from build123d import *

# Parameters (mm, degrees)
SKETCH_1_W          = 40.75
SKETCH_1_H          = 20.2
EXTRUDE_1_DEPTH     = 20.65
SHELL_1_T           = -1.65
SKETCH_2_W          = 40.75
SKETCH_2_H          = 20.2
EXTRUDE_2_DEPTH     = 1
EXTRUDE_3_DEPTH     = 1.23
SKETCH_4_R          = 3.95
SKETCH_4_R_2        = 0.8
EXTRUDE_4_DEPTH     = 5
EXTRUDE_5_DEPTH     = 2
SKETCH_6_R          = 2.9
SKETCH_6_R_2        = 2.4
EXTRUDE_6_DEPTH     = 4
SKETCH_7_W          = 38.95
SKETCH_7_H          = 18.4
CUT_EXTRUDE_2_DEPTH = 2.6
SKETCH_9_R          = 1.4
EXTRUDE_7_DEPTH     = 17.05
CUT_EXTRUDE_START   = -19.28
SKETCH_8_R          = 1
CUT_EXTRUDE_3_DEPTH = 19.28


with BuildPart() as part:
    # Эскиз1 → Бобышка-Вытянуть1 (new body)
    with BuildSketch(Plane(origin=(0, 0, 0), x_dir=(1, 0, 0), z_dir=(0, 1, 0))):
        Rectangle(SKETCH_1_W, SKETCH_1_H)
    extrude(amount=EXTRUDE_1_DEPTH)

    # Оболочка1
    shell_1_openings = [part.faces().sort_by_distance(p)[0] for p in [
        (0, 20.65, 0),
        (0, 0, 0),
    ]]
    offset(amount=SHELL_1_T, openings=shell_1_openings, kind=Kind.INTERSECTION)

    # Эскиз2 → Бобышка-Вытянуть2 (add)
    with BuildSketch(Plane(origin=(0, 20.65, 0), x_dir=(1, 0, 0), z_dir=(0, 1, 0))):
        Rectangle(SKETCH_2_W, SKETCH_2_H)
    extrude(amount=-EXTRUDE_2_DEPTH)

    # Эскиз3 → Бобышка-Вытянуть3 (add)
    with BuildSketch(Plane(origin=(0, 20.65, 0), x_dir=(1, 0, 0), z_dir=(0, 1, 0))):
        Polygon((-19.375, -9.1), (-3, -9.1), (-3, -7.8), (-18.075, -7.8), (-18.075, 7.8), (-3, 7.8), (-3, 9.1), (-19.375, 9.1), align=None)
        Polygon((19.375, -9.1), (19.375, 9.1), (3, 9.1), (3, 7.8), (18.075, 7.8), (18.075, -7.8), (3, -7.8), (3, -9.1), align=None)
    extrude(amount=EXTRUDE_3_DEPTH)

    # Эскиз4 → Бобышка-Вытянуть4 (add)
    with BuildSketch(Plane(origin=(0, 20.65, 0), x_dir=(1, 0, 0), z_dir=(0, 1, 0))):
        with Locations(Location((-10.325, 0, 0), (0, 0, 90))):
            Circle(SKETCH_4_R)
        with Locations(Location((-10.325, 0, 0), (0, 0, 270))):
            Circle(SKETCH_4_R_2, mode=Mode.SUBTRACT)
    extrude(amount=EXTRUDE_4_DEPTH)

    # Эскиз5 → Бобышка-Вытянуть5 (add)
    with BuildSketch(Plane(origin=(0, 20.65, 0), x_dir=(1, 0, 0), z_dir=(0, 1, 0))):
        with BuildLine():
            Line((7.475, 2.607680962), (7.475, -2.607680962))
            ThreePointArc((7.475, -2.607680962), (14.275, 0), (7.475, 2.607680962))
        make_face()
    extrude(amount=EXTRUDE_5_DEPTH)

    # Эскиз6 → Бобышка-Вытянуть6 (add)
    with BuildSketch(Plane(origin=(0, 22.65, 0), x_dir=(1, 0, 0), z_dir=(0, 1, 0))):
        with Locations(Location((10.375, 0, 0), (0, 0, 180))):
            Circle(SKETCH_6_R)
        with Locations(Location((10.375, 0, 0), (0, 0, 270))):
            Circle(SKETCH_6_R_2, mode=Mode.SUBTRACT)
    extrude(amount=EXTRUDE_6_DEPTH)

    # Эскиз7 → Вырез-Вытянуть2 (cut)
    with BuildSketch(Plane.XZ):
        Rectangle(SKETCH_7_W, SKETCH_7_H)
    extrude(amount=-CUT_EXTRUDE_2_DEPTH, mode=Mode.SUBTRACT)

    # Эскиз9 → Бобышка-Вытянуть7 (add)
    with BuildSketch(Plane.XZ.offset(-19.65)):
        with Locations((-18.25, 7.55)):
            Circle(SKETCH_9_R)
        with Locations((-18.25, -7.55)):
            Circle(SKETCH_9_R)
        with Locations((18.25, -7.55)):
            Circle(SKETCH_9_R)
        with Locations((18.25, 7.55)):
            Circle(SKETCH_9_R)
    extrude(amount=EXTRUDE_7_DEPTH)

    # Эскиз8 → Вырез-Вытянуть3 (cut)
    with BuildSketch(Plane(origin=(0, 21.88, 0), x_dir=(1, 0, 0), z_dir=(0, 1, 0)).offset(CUT_EXTRUDE_START)):
        with Locations(Location((-18.25, 7.55, 0), (0, 0, 270))):
            Circle(SKETCH_8_R)
        with Locations(Location((18.25, 7.55, 0), (0, 0, 270))):
            Circle(SKETCH_8_R)
        with Locations(Location((18.25, -7.55, 0), (0, 0, 270))):
            Circle(SKETCH_8_R)
        with Locations(Location((-18.25, -7.55, 0), (0, 0, 270))):
            Circle(SKETCH_8_R)
    extrude(amount=CUT_EXTRUDE_3_DEPTH, mode=Mode.SUBTRACT)


solid = part.part
Input: part model. Units: mm. Frame: model coordinates. A direction names the side the tool comes from. Give positions to 0.01 mm unless a question says otherwise; leave off trailing zeros. Write each loop counter-clockwise with the first axis right and the second up, starting at its lowest first coordinate (ties: lowest second). Pieces come first, ordered by that corner, then holes.
Q1. First-contact query: P1, Ø12, axis at x = -10, z = -2, coming from the -Y side; P2, Ø5, axis at x = -16, z = 7, coming from the -Y side; P3, Ø1, axis at x = 13, y = 21.5, coming from the -Z side; P4, Ø1.4, axis at x = 14.5, y = 21.5, coming from the +Z side. Flat tips, straight axial feed; report the tip coordinate or a pass-through.
Q2. Section C-C, the plane y = 24.5. Output: boundary loops of the cut face in (x, z) (3 decimals), plus the area to 3 significant figures.
Q3. Material intervals for probe 1 along Z at (x, y) = (-18.25, 13.25); probe 2 along X at (y, z) = (9.75, -7.55) (3 decimals); probe 3 along X at (y, z) = (8.5, 2.5) (3 decimals), sorted ascending.
Q4. Section A-A, the plane y = 19. Output: boundary loops of the cut face in (x, z) (3 decimals).
Q5. Section B-B, the plane x = 4. Output: boundary loops of the cut face in (y, z).
Q6. Section D-D, the plane x = -7. Output: boundary loops of the cut face in (y, z).
Q7. Set-up query: faces 1 (the face through (18.4, 21.88, -0.7)), 2 (the face through (3, 21, 8)), 3 (the face through (12, 26.65, 2)), 4 (the face through (-11.1, 23.1, -0.2)), 5 (the face through (0, 1, -9.2)). Return all of +Z, -Z, +X, -X, +Y, -Y with unobstructed straight access to the full face (end or side cutting, diameter ignored); none if empty.
Q8. Pull-direction query (X, two-part tool) for faces 6 (the face through (3, 21, -8)), 7 (the face through (20.375, 10, 0)), 8 (the face through (17.088, 11.244, 6.77)), 9 (the face through (-20.375, 10, 0)); classes: pulls with the +X half, pulls with the -X half, needs draft (parallel to the pull), parting line crosses it, or undercut.
Filled in:
1. P1: stops at y = 19.65
1. P2: stops at y = 0
1. P3: stops at z = -9.1
1. P4: stops at z = 9.1
2. outline: circle Ø7.9 at (-10.325, 0); circle Ø5.8 at (10.375, 0); hole circle Ø1.6 at (-10.325, 0); hole circle Ø4.8 at (10.375, 0)
2. area: 55.3 mm2
3. probe 1: z = -10.1 to -8.55, -6.55 to -6.15, 6.15 to 6.55, 8.55 to 10.1
3. probe 2: x = -20.375 to -19.25, -17.25 to -16.85, 16.85 to 17.25, 19.25 to 20.375
3. probe 3: x = -20.375 to -18.725, 18.725 to 20.375
4. outline: (-20.375, -10.1) - (20.375, -10.1) - (20.375, 10.1) - (-20.375, 10.1) - close; hole circle Ø2 at (-18.25, -7.55); hole circle Ø2 at (-18.25, 7.55); hole (-18.725, -6.233) arc R1.4 cw to (-17.178, -8.45) - (17.178, -8.45) arc R1.4 cw to (18.725, -6.233) - (18.725, 6.233) arc R1.4 cw to (17.178, 8.45) - (-17.178, 8.45) arc R1.4 cw to (-18.725, 6.233) - close; hole circle Ø2 at (18.25, -7.55); hole circle Ø2 at (18.25, 7.55)
5. outline: (0, -10.1) - (20.65, -10.1) - (20.65, -9.1) - (21.88, -9.1) - (21.88, -7.8) - (20.65, -7.8) - (20.65, 7.8) - (21.88, 7.8) - (21.88, 9.1) - (20.65, 9.1) - (20.65, 10.1) - (0, 10.1) - (0, 9.2) - (2.6, 9.2) - (2.6, 8.45) - (19.65, 8.45) - (19.65, -8.45) - (2.6, -8.45) - (2.6, -9.2) - (0, -9.2) - close
6. outline: (0, -10.1) - (20.65, -10.1) - (20.65, -9.1) - (21.88, -9.1) - (21.88, -7.8) - (20.65, -7.8) - (20.65, -2.13) - (25.65, -2.13) - (25.65, 2.13) - (20.65, 2.13) - (20.65, 7.8) - (21.88, 7.8) - (21.88, 9.1) - (20.65, 9.1) - (20.65, 10.1) - (0, 10.1) - (0, 9.2) - (2.6, 9.2) - (2.6, 8.45) - (19.65, 8.45) - (19.65, -8.45) - (2.6, -8.45) - (2.6, -9.2) - (0, -9.2) - close
7. face 1: +X, +Y
7. face 2: +Z, -Z, +Y
7. face 3: +Z, -Z, +X, -X, +Y
7. face 4: +Y
7. face 5: -Y
8. face 6: undercut
8. face 7: pulls with the +X half
8. face 8: undercut
8. face 9: pulls with the -X half
